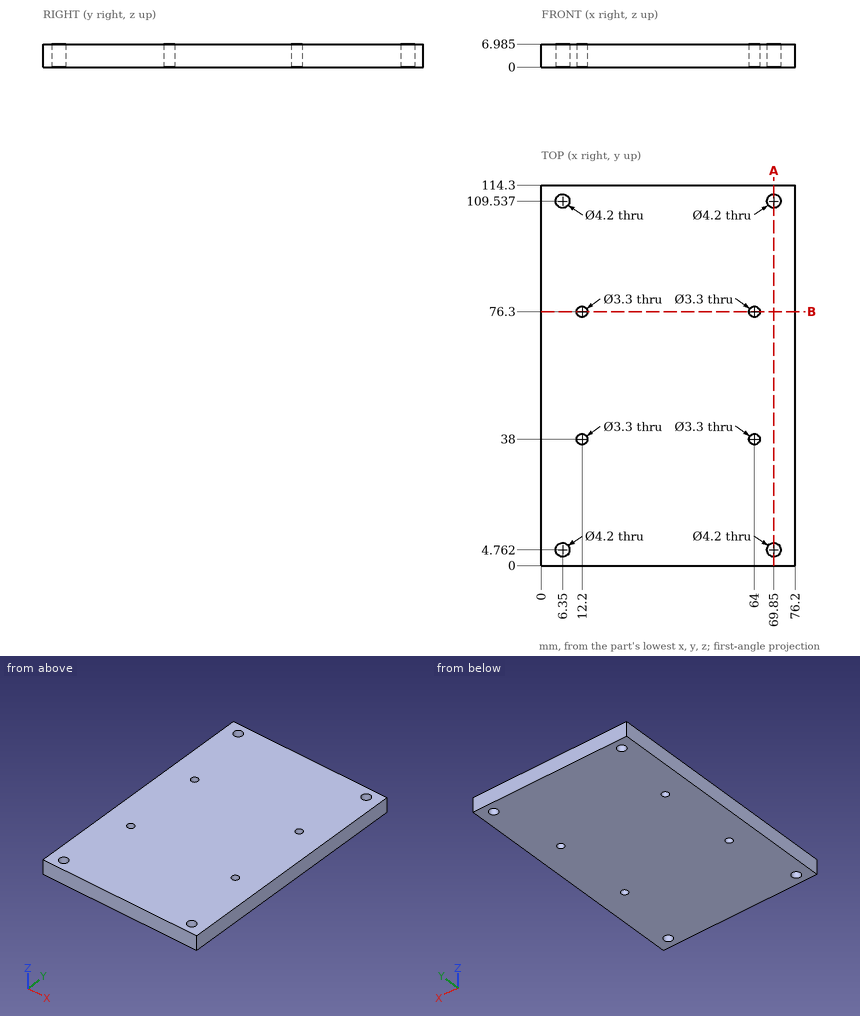
Geometry check sheet. Reference: drawing and pictorial views, mm from the part's lowest x, y, z. Round coordinates to 2 decimals unless told otherwise and drop trailing zeros. Loops run counter-clockwise (first coordinate to the right, second up) from the corner with the lowest first, then second, coordinate; pieces in that order, holes last. Notation, with made-up numbers: M 57.25,85 L 71.25,85 A21 ccw 71.25,95 Z; hole C 79,-11.75 d4. An arc over 180 degrees is marked long. Return JSON: item names as keys, results as strings. Group by question number.
(1) Scan lines: line 1 along Y through (x, z) = (64, 3.5); line 2 along Y through (x, z) = (6.35, 4.5); line 3 along X through (y, z) = (76.3, 2.5). Record each from-to range of solid material in increasing order. Write a range as [from, to].
(2) Go/stop test with a flat-tipped pin: pin 1 (3.5 mm diameter, centred on x = 69.85, y = 109.54, fed in from +Z). Record where the tip stops, or that it passes through.
(3) Section check A-A, the plane x = 69.85. Enter the section's corners in (y, z) (1 decimal).
(4) Section check B-B, the plane y = 76.3. Give the number of separate pieces and of enclosed holes in the cut face, and give its area (3 significant figures).
Data:
{
 "1": {"line 1": "[0, 36.35], [39.65, 74.65], [77.95, 114.3]", "line 2": "[0, 2.66], [6.86, 107.44], [111.64, 114.3]", "line 3": "[0, 10.55], [13.85, 62.35], [65.65, 76.2]"},
 "2": {"pin 1": "through"},
 "3": {"outline": "M 0,0 L 2.7,0 L 2.7,7 L 0,7 Z; M 6.9,0 L 107.4,0 L 107.4,7 L 6.9,7 Z; M 111.6,0 L 114.3,0 L 114.3,7 L 111.6,7 Z"},
 "4": {"separate pieces": "3", "enclosed holes": "0", "area": "486 mm²"}
}
